```python
from build123d import *

# Parameters (mm, degrees)
SKETCH1_W                = 304.8
SKETCH1_H                = 304.8
BOSS_EXTRUDE1_DEPTH      = 38.1
SKETCH2_R                = 6.5151
HAAS_T_SLOT_HOLES_DEPTH  = 219.867836833
SKETCH3_R                = 9.779
HAAS_COUNTER_BORES_DEPTH = 22.225


with BuildPart() as part:
    # Sketch1 → Boss-Extrude1 (new body)
    with BuildSketch(Plane.XY):
        Rectangle(SKETCH1_W, SKETCH1_H)
    extrude(amount=BOSS_EXTRUDE1_DEPTH)

    # Sketch2 → HAAS T-Slot Holes (cut, through all)
    with BuildSketch(Plane.XY.offset(38.1)):
        with Locations((-127, 101.6)):
            Circle(SKETCH2_R)
        with Locations((127, 101.6)):
            Circle(SKETCH2_R)
        with Locations((127, -101.6)):
            Circle(SKETCH2_R)
        with Locations((-127, -101.6)):
            Circle(SKETCH2_R)
        Circle(SKETCH2_R)
    extrude(amount=-HAAS_T_SLOT_HOLES_DEPTH, mode=Mode.SUBTRACT)

    # Sketch3 → HAAS Counter Bores (cut)
    with BuildSketch(Plane.XY.offset(38.1)):
        with Locations((-127, 101.6)):
            Circle(SKETCH3_R)
        with Locations((127, 101.6)):
            Circle(SKETCH3_R)
        Circle(SKETCH3_R)
        with Locations((127, -101.6)):
            Circle(SKETCH3_R)
        with Locations((-127, -101.6)):
            Circle(SKETCH3_R)
    extrude(amount=-HAAS_COUNTER_BORES_DEPTH, mode=Mode.SUBTRACT)


solid = part.part
```
Could you check a few things on this model? Use its own coordinates, in mm. A direction names the side the tool comes from. Round coordinates to 2 decimals unless told otherwise and drop trailing zeros. Write each loop counter-clockwise with the first axis right and the second up, starting at its lowest first coordinate (ties: lowest second). Pieces come first, ordered by that corner, then holes.
(1) For pin 1 (11.5 mm diameter, centred on x = -127, y = -101.6, fed in from -Z), with a flat end and sliding along its axis, tell me the tip position at first contact or that it passes through.
Findings below:
pin 1: passes through
(2) Which directions (+Z, -Z, +X, -X, +Y, -Y) give clear straight access to the entire face, cutting with the end or side of a thin tool? Please do faces 4 (the face through (-125, 95, 15.875)), 5 (the face through (-2, -152.4, 19)).
Findings below:
face 4: +Z
face 5: +Z, -Z, +X, -X, -Y
(3) Suppose I cut it at D-D on y = -101.6. Write out the boundary of the cut face in (x, z) (3 decimals).
Findings below:
outline: (-152.4, 0) - (-133.515, 0) - (-133.515, 15.875) - (-136.779, 15.875) - (-136.779, 38.1) - (-152.4, 38.1) - close; (-120.485, 0) - (120.485, 0) - (120.485, 15.875) - (117.221, 15.875) - (117.221, 38.1) - (-117.221, 38.1) - (-117.221, 15.875) - (-120.485, 15.875) - close; (133.515, 0) - (152.4, 0) - (152.4, 38.1) - (136.779, 38.1) - (136.779, 15.875) - (133.515, 15.875) - close
(4) Suppose I cut it at C-C on x = 127. Write out the boundary of the cut face in (y, z) (3 decimals), and give its area (3 significant figures).
Findings below:
outline: (-152.4, 0) - (-108.115, 0) - (-108.115, 15.875) - (-111.379, 15.875) - (-111.379, 38.1) - (-152.4, 38.1) - close; (-95.085, 0) - (95.085, 0) - (95.085, 15.875) - (91.821, 15.875) - (91.821, 38.1) - (-91.821, 38.1) - (-91.821, 15.875) - (-95.085, 15.875) - close; (108.115, 0) - (152.4, 0) - (152.4, 38.1) - (111.379, 38.1) - (111.379, 15.875) - (108.115, 15.875) - close
area: 10,300 mm2
(5) Thinking about a two-plate mould opening in X: for faces 1 (the face through (-152.4, -2, 19)), 2 (the face through (-123.498, 107.094, 8.049)), 3 (the face through (152.4, -2, 19)), which applies, +X half, -X half, draft (parallel to the pull), parting line (faces both ways), or undercut?
Findings below:
face 1: -X half
face 2: undercut
face 3: +X half
(6) If I drill on probe 1 along Y at (x, z) = (-127, 12.25); probe 2 along Y at (x, z) = (-127, 28); probe 3 along X at (y, z) = (101, 12), over which ranges is the centre line in solid material (lowest first)?
Findings below:
probe 1: y = -152.4 to -108.12, -95.08 to 95.08, 108.12 to 152.4
probe 2: y = -152.4 to -111.38, -91.82 to 91.82, 111.38 to 152.4
probe 3: x = -152.4 to -133.49, -120.51 to 120.51, 133.49 to 152.4
(7) Suppose I cut it at A-A on x = 0. Write out the boundary of the cut face in (y, z) (3 decimals).
Findings below:
outline: (-152.4, 0) - (-6.515, 0) - (-6.515, 15.875) - (-9.779, 15.875) - (-9.779, 38.1) - (-152.4, 38.1) - close; (6.515, 0) - (152.4, 0) - (152.4, 38.1) - (9.779, 38.1) - (9.779, 15.875) - (6.515, 15.875) - close
